from build123d import *

# Parameters (mm, degrees)
BOSS_EXTRUDE1_DEPTH      = 3
BOSS_EXTRUDE1_DEPTH_BACK = 3
BOSS_EXTRUDE2_DEPTH      = 3
BOSS_EXTRUDE2_DEPTH_BACK = 3
BOSS_EXTRUDE3_DEPTH      = 1.5
BOSS_EXTRUDE3_DEPTH_BACK = 1.5
SKETCH3_W                = 3
SKETCH3_H                = 52


with BuildPart() as part:
    # Sketch1 → Boss-Extrude1 (new, two sides: drawn at the far end of the back side and taken through both)
    with BuildSketch(Plane(origin=(0, 0, 0), x_dir=(0, 0, -1), z_dir=(1, 0, 0)).offset(-BOSS_EXTRUDE1_DEPTH_BACK)):
        with BuildLine():
            Line((-7.25, 0), (-4.25, 0))
            ThreePointArc((-4.25, 0), (0, 4.25), (4.25, 0))
            ThreePointArc((4.25, 0), (4.213640661, -0.554736317), (4.105184762, -1.099980942))
            Line((4.105184762, -1.099980942), (7.002962241, -1.876438077))
            ThreePointArc((7.002962241, -1.876438077), (7.187975245, -0.946314894), (7.25, 0))
            ThreePointArc((7.25, 0), (0, 7.25), (-7.25, 0))
        make_face()
        with BuildLine():
            Line((7.002962241, -1.876438077), (4.105184762, -1.099980942))
            ThreePointArc((4.105184762, -1.099980942), (5.165844934, -2.937098249), (7.002962241, -1.876438077))
        make_face()
        with BuildLine():
            ThreePointArc((-4.105184762, -1.099980942), (-4.213640661, -0.554736317), (-4.25, 0))
            Line((-4.25, 0), (-7.25, 0))
            ThreePointArc((-7.25, 0), (-7.187975245, -0.946314894), (-7.002962241, -1.876438077))
            Line((-7.002962241, -1.876438077), (-5.554073501, -1.488209509))
            Line((-5.554073501, -1.488209509), (-4.105184762, -1.099980942))
        make_face()
        with BuildLine():
            ThreePointArc((-7.002962241, -1.876438077), (-5.165844934, -2.937098249), (-4.105184762, -1.099980942))
            Line((-4.105184762, -1.099980942), (-5.554073501, -1.488209509))
            Line((-5.554073501, -1.488209509), (-7.002962241, -1.876438077))
        make_face()
    extrude(amount=BOSS_EXTRUDE1_DEPTH + BOSS_EXTRUDE1_DEPTH_BACK)

    # Sketch2 → Boss-Extrude2 (add, two sides: drawn at the far end of the back side and taken through both)
    with BuildSketch(Plane(origin=(0, 0, 0), x_dir=(0, 0, -1), z_dir=(1, 0, 0)).offset(-BOSS_EXTRUDE2_DEPTH_BACK)):
        Polygon((0, 7.25), (0, 5.25), (3, 5.25), (3, 58.25), (0, 58.25), align=None)
    extrude(amount=BOSS_EXTRUDE2_DEPTH + BOSS_EXTRUDE2_DEPTH_BACK)

    # Sketch3 → Boss-Extrude3 (add, two sides: drawn at the far end of the back side and taken through both)
    with BuildSketch(Plane(origin=(0, 0, 0), x_dir=(0, 0, -1), z_dir=(1, 0, 0)).offset(-BOSS_EXTRUDE3_DEPTH_BACK)):
        with Locations((-1.5, 32.25)):
            Rectangle(SKETCH3_W, SKETCH3_H)
    extrude(amount=BOSS_EXTRUDE3_DEPTH + BOSS_EXTRUDE3_DEPTH_BACK)


solid = part.part
Read the model definition and answer for the solid it produces. Units are mm, in the model's axes. A direction names the side the tool comes from. Round coordinates to 2 decimals unless told otherwise and drop trailing zeros. Write each loop counter-clockwise with the first axis right and the second up, starting at its lowest first coordinate (ties: lowest second). Pieces come first, ordered by that corner, then holes.
Q1. A tool of negligible diameter and unlimited length cuts with its end or side. For faces 1 (the face through (2, 33, 0)), 2 (the face through (0, 58.25, -1)), 3 (the face through (-1.5, 33, 2)), 4 (the face through (-3, 23, -1)), 5 (the face through (0, 32, -3)), from which of +Z, -Z, +X, -X, +Y, -Y can it reach the whole face along a straight path? Write none if from no direction.
Values:
face 1: +Z, +X, +Y
face 2: +Z, -Z, +X, -X, +Y
face 3: +Z, -X, +Y
face 4: +Z, -Z, -X, +Y, -Y
face 5: -Z, +X, -X, +Y
Q2. The mould has two halves that part along Z. Classify faces 6 (the face through (0, 32, 3)), 7 (the face through (-0.042, -2.945, 5.198)), 8 (the face through (-0.042, -2.928, -5.134)), 9 (the face through (3, 23, -1)): released by +Z, released by -Z, zero draft, split by the parting line, or undercut.
Values:
face 6: released by +Z
face 7: undercut
face 8: undercut
face 9: zero draft
Q3. Straight lines are drawn through the part: line 1 (Z direction, x = 0.85, y = 50.5); line 2 (Z direction, x = 2.7, y = 43); line 3 (X direction, y = 31, z = 0.75). For each, find the intervals that lie inside material, in ascending order.
Values:
line 1: z = -3 to 3
line 2: z = -3 to 0
line 3: x = -1.5 to 1.5
Q4. Find section A-A on x = -0.1. Determine the outline of the cut face in (y, z).
Values:
outline: (-1.88, -7) arc R7.25 ccw to (6.6, -3) - (58.25, -3) - (58.25, 3) - (6.6, 3) arc R7.25 ccw to (-1.88, 7) arc R1.5 ccw to (-1.1, 4.11) arc R4.25 cw (long way) to (-1.1, -4.11) arc R1.5 ccw to start
Q5. Find section C-C on z = 5.75. Determine the outline of the cut face in (x, y), and give its area (3 significant figures).
Values:
outline: (-3, -2.98) - (3, -2.98) - (3, 4.42) - (-3, 4.42) - close
area: 44.3 mm2
Q6. Flat-ended cylindrical pins translate along their axes: P1, Ø0.9, axis at y = 35.5, z = 2, coming from the +X side; P2, Ø3.5, axis at y = 27, z = 2, coming from the -X side; P3, Ø1.8, axis at x = -1, y = 23, coming from the -Z side. Find the tip coordinate at first contact, or state that the pin passes through.
Values:
P1: stops at x = 1.5
P2: stops at x = -1.5
P3: stops at z = -3
Q7. Find section B-B on y = 54. Determine the outline of the cut face in (x, z), and give its area (3 significant figures).
Values:
outline: (-3, -3) - (3, -3) - (3, 0) - (1.5, 0) - (1.5, 3) - (-1.5, 3) - (-1.5, 0) - (-3, 0) - close
area: 27.0 mm2
